from build123d import *

# Parameters (mm, degrees)
F1_DEPTH = 3.429
F2_R     = 0.381


# Not quite as in the source:
# - ends of sketch curves that miss each other by under 0.0002 mm in the source are joined


with BuildPart() as f1:
    # F0 (on Front) → F1 (new body)
    with BuildSketch(Plane.XZ):
        with BuildLine():
            ThreePointArc((-523.3072592, 342.1259096), (-528.0697592, 346.8884096), (-523.3072592, 351.6509096))
            ThreePointArc((-523.3072592, 351.6509096), (-500.8987443088, 356.1961233076), (-482.0322439898, 369.1133948419))
            Line((-482.0322439898, 369.1133948419), (-505.5272592, 369.1134096))
            Line((-505.5272592, 369.1134096), (-505.5272592, 372.2884096))
            Line((-505.5272592, 372.2884096), (-523.3072592, 372.2884096))
            Line((-523.3072592, 372.2884096), (-523.3072592, 369.1134096))
            Line((-523.3072592, 369.1134096), (-536.0072592, 369.1134096))
            ThreePointArc((-536.0072592, 369.1134096), (-541.5868750184, 355.6430254184), (-555.0572592, 350.0634096))
            Line((-555.0572592, 350.0634096), (-555.0572592, 321.4884096))
            Line((-555.0572592, 321.4884096), (-542.3572592, 321.4884096))
            Line((-542.3572592, 321.4884096), (-451.219951, 347.675962))
            ThreePointArc((-451.219951, 347.675962), (-444.5824868492, 352.2417976203), (-442.0272592, 359.882059))
            Line((-442.0272592, 359.882059), (-442.0272592, 363.0174096))
            Line((-442.0272592, 363.0174096), (-293.4372592, 363.0174096))
            Line((-293.4372592, 363.0174096), (-293.4372592, 369.1134096))
            Line((-293.4372592, 369.1134096), (-306.1372592, 369.1134096))
            Line((-306.1372592, 369.1134096), (-306.1372592, 372.2884096))
            Line((-306.1372592, 372.2884096), (-323.9172592, 372.2884096))
            Line((-323.9172592, 372.2884096), (-323.9172592, 369.1134096))
            Line((-323.9172592, 369.1134096), (-443.2972592, 369.1134096))
            Line((-443.2972592, 369.1134096), (-443.2972592, 372.2884096))
            Line((-443.2972592, 372.2884096), (-461.0772592, 372.2884096))
            Line((-461.0772592, 372.2884096), (-461.0772592, 369.1134096))
            Line((-461.0772592, 369.1134096), (-462.9822592, 369.1134096))
            ThreePointArc((-462.9822592, 369.1134096), (-463.9484088233, 364.9334927075), (-466.650858723, 361.601539097))
            ThreePointArc((-466.650858723, 361.601539097), (-493.3520932085, 347.1307312076), (-523.3072592, 342.1259096))
        make_face()
    extrude(amount=F1_DEPTH)

    # F2
    f2_edges = [f1.edges().sort_by_distance(p)[0] for p in [
        (-482.032244, -1.7145, 369.113395),
        (-461.077259, -1.7145, 372.28841),
        (-461.077259, -1.7145, 369.11341),
        (-462.982259, -1.7145, 369.11341),
        (-505.527259, -1.7145, 372.28841),
        (-523.307259, -1.7145, 372.28841),
        (-523.307259, -1.7145, 369.11341),
        (-536.007259, -1.7145, 369.11341),
        (-505.527259, -1.7145, 369.11341),
        (-555.057259, -1.7145, 350.06341),
        (-443.297259, -1.7145, 369.11341),
        (-443.297259, -1.7145, 372.28841),
        (-323.917259, -1.7145, 372.28841),
        (-306.137259, -1.7145, 372.28841),
        (-306.137259, -1.7145, 369.11341),
        (-323.917259, -1.7145, 369.11341),
        (-293.437259, -1.7145, 369.11341),
        (-293.437259, -1.7145, 363.01741),
        (-542.357259, -1.7145, 321.48841),
        (-555.057259, -1.7145, 321.48841),
    ]]
    fillet(f2_edges, radius=F2_R)


solid = f1.part
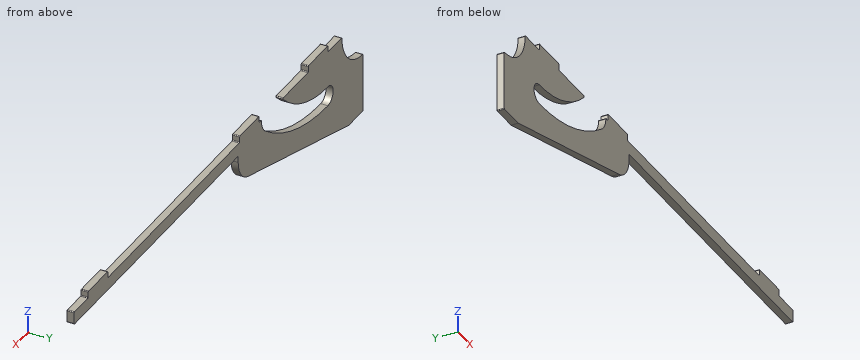
Input: part model. Units: mm. Frame: model coordinates. Round coordinates to 2 decimals unless told otherwise and drop trailing zeros. Loops run counter-clockwise (first coordinate to the right, second up) from the corner with the lowest first, then second, coordinate; pieces in that order, holes last. Notation, with made-up numbers: M 45,-35.75 L 51,-35.75 A28 ccw 51,-3.75 Z; hole C 9,-20.5 d8. An arc over 180 degrees is marked long. Answer as CSV lines item,"result". Start each with the question number.
(1) Section A-A, the plane x = -514. Output: boundary loops of the cut face in (y, z).
(2) Line query: line 1 (X direction, y = -3.3, z = 369); line 2 (Z direction, x = -412, y = -2.3); line 3 (Z direction, x = -502.5, y = -0.5). Output: solid intervals per line, ascending. Write a range as [from, to].
(3) Section B-B, the plane x = -312.5. Output: boundary loops of the cut face in (y, z), plus the area to 3 significant figures.
(4) First-contact query: pin 1 (0.9 mm diameter, centred on x = -462, y = -2, fed in from +Z); pin 2 (1.9 mm diameter, centred on y = -1.5, z = 370.5, fed in from +X); pin 3 (1.7 mm diameter, centred on x = -365.5, y = -2.5, fed in from -Z); pin 4 (4 mm diameter, centred on x = -477, z = 337, fed in from +Y). Flat tips, straight axial feed; report the tip coordinate or a pass-through.
(5) Section C-C, the plane x = -446. Output: boundary loops of the cut face in (y, z), plus the area to 3 significant figures.
Values found:
1,outline,"M -3.43,329.64 L 0,329.64 L 0,342.6 L -3.43,342.6 Z; M -3.43,352.41 L 0,352.41 L 0,372.29 L -3.43,372.29 Z"
2,line 1,"x = [-535.9, -482.67], [-462.88, -293.55]"
2,line 2,"z = [363.02, 369.11]"
2,line 3,"z = [332.94, 344.51], [355.55, 369.11]"
3,outline,"M -3.43,363.02 L 0,363.02 L 0,372.29 L -3.43,372.29 Z"
3,area,"31.8 mm²"
4,pin 1,"stops at z = 369.11"
4,pin 2,"stops at x = -306.14"
4,pin 3,"stops at z = 363.02"
4,pin 4,"passes through"
5,outline,"M -3.43,350.66 L 0,350.66 L 0,372.29 L -3.43,372.29 Z"
5,area,"74.2 mm²"
